```python
from build123d import *

# Parameters (mm, degrees)
EXTRUDE_1_DEPTH     = 10
SKETCH_2_R          = 3
CUT_EXTRUDE_1_DEPTH = 25


with BuildPart() as part:
    # Эскиз1 → Вытянуть1 (new body)
    with BuildSketch(Plane(origin=(0, 0, 0), x_dir=(0, 0, -1), z_dir=(1, 0, 0))):
        Polygon((-19.99990009, 63.483695787), (-5.430696524, 94.358841013), (-5.430696524, 136.453197444), (31.353949284, 136.453197444), (31.353949284, 81.897126676), (20.00009991, 58.395614664), (20.00009991, -30.143863535), (-19.99990009, -30.143863535), align=None)
    extrude(amount=EXTRUDE_1_DEPTH)

    # Эскиз2 → Вырез-Вытянуть1 (cut)
    with BuildSketch(Plane.ZY):
        with Locations((-12.96162638, 126.453197444)):
            Circle(SKETCH_2_R)
    extrude(amount=-CUT_EXTRUDE_1_DEPTH, mode=Mode.SUBTRACT)


solid = part.part
```
Work out the finished part from the listing and answer in its coordinate system (mm). A direction names the side the tool comes from. Coordinates: 2 decimals unless noted, no trailing zeros. Write each loop counter-clockwise with the first axis right and the second up, starting at its lowest first coordinate (ties: lowest second). Pieces come first, ordered by that corner, then holes.
Q1. A cutting plane is placed at A-A, the plane x = 2.5. Give the vertices of the cut face in (y, z).
Q2. A cutting plane is placed at B-B, the plane y = 103.5. Give the vertices of the cut face in (x, z), then the cut area to 3 significant figures.
Q3. A cutting plane is placed at C-C, the plane z = 16. Give the vertices of the cut face in (x, y).
Q4. Which of the six approach directions +Z, -Z, +X, -X, +Y, -Y give full straight-line access (tool end or side, diameter ignored) to faces 4 (the face through (5, 15, -20)), 5 (the face through (5, 115, 5.431)), 6 (the face through (5, 136.453, -13))?
Q5. Determine the mould class of faces 1 (the face through (4.93, 129.428, -13.352)), 2 (the face through (10, 54, -6)), 3 (the face through (5, 110, -31.354)) for opening direction Z: released by +Z, released by -Z, zero draft, split by the parting line, or undercut.
Q6. Each of these flat-tipped pins is pushed along its axis until it touches: pin 1 Ø2 at (y, z) = (64.5, 0.5) entering from -X; pin 2 Ø6 at (x, y) = (4.5, 55) entering from -Z; pin 3 Ø5 at (x, y) = (6.5, 120) entering from +Z. Where does it stop, or does it pass through?
Q7. Find the intervals of material crossed by line 1 (Z direction, x = 4.5, y = 103); line 2 (Z direction, x = 2.5, y = 28.5); line 3 (Y direction, x = 3.75, z = -11), in increasing order.
Findings below:
1. outline: (-30.14, -20) - (58.4, -20) - (81.9, -31.35) - (136.45, -31.35) - (136.45, 5.43) - (94.36, 5.43) - (63.48, 20) - (-30.14, 20) - close; hole circle Ø6 at (126.45, -12.96)
2. outline: (0, -31.35) - (10, -31.35) - (10, 5.43) - (0, 5.43) - close
2. area: 368 mm2
3. outline: (0, -30.14) - (10, -30.14) - (10, 71.96) - (0, 71.96) - close
4. face 4: -Z, +X, -X, -Y
4. face 5: +Z, +X, -X, +Y
4. face 6: +Z, -Z, +X, -X, +Y
5. face 1: undercut
5. face 2: zero draft
5. face 3: released by -Z
6. pin 1: stops at x = 0
6. pin 2: stops at z = -20
6. pin 3: stops at z = 5.43
7. line 1: z = -31.35 to 5.43
7. line 2: z = -20 to 20
7. line 3: y = -30.14 to 124.18, 128.72 to 136.45
